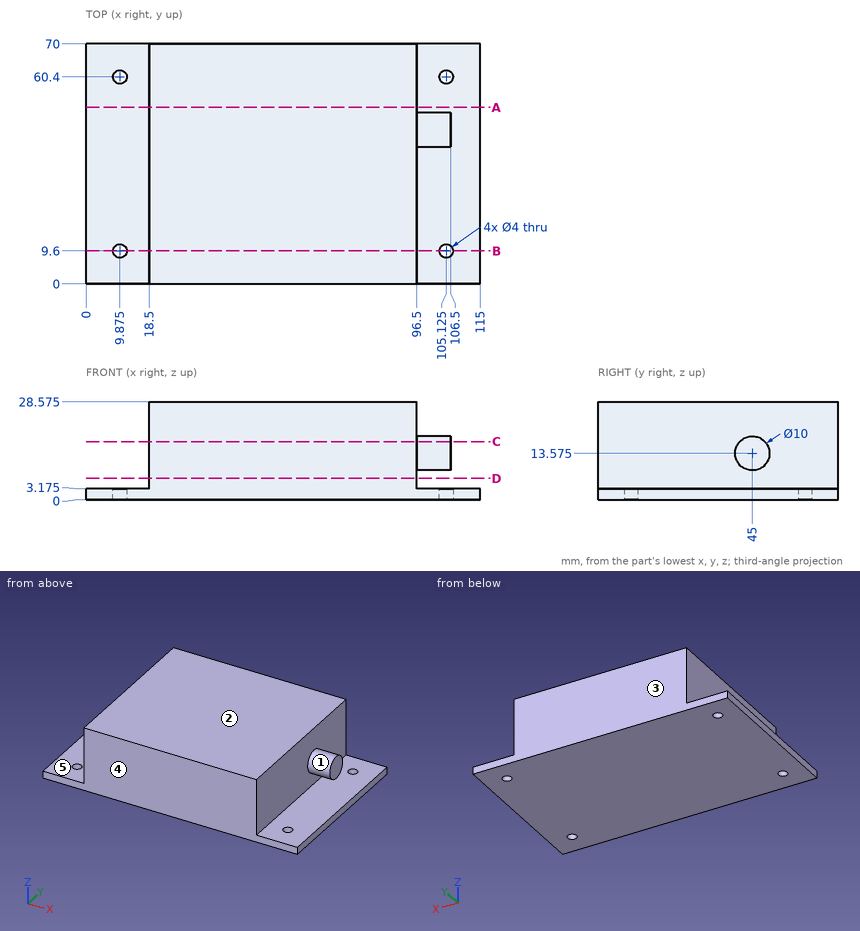
Here's the drawing with two shaded views (mm, measured from the low corner). I have some questions. A direction names the side the tool comes from. Give positions to 0.01 mm unless a question says otherwise; leave off trailing zeros. Order: outer loops, then holes, each group sorted by start corner. A loop starts at its lowest first (then second) coordinate and runs counter-clockwise, first axis right, second up. Notation, with made-up numbers: (81, 55.5) - (136, 55.5) arc R7 ccw to (136, 67.5) - close; hole circle Ø4 at (50, 69.25). An arc over 180 degrees is marked (long way). Use a Markdown table: item, result. Add a question column.
Q1. If we section it at A-A on y = 51.5: Write out the boundary of the cut face in (x, z) (3 decimals).
Q2. If we section it at B-B on y = 9.6: Write out the boundary of the cut face in (x, z) (3 decimals).
Q3. On a 3-axis mill with a long thin cutter (end or side, diameter ignored), from which of +Z, -Z, +X, -X, +Y, -Y can I reach the whole of each face in a straight line? I mean the marked faces 4 and 5. Say none if no direction works.
Q4. Please list where these lines run through material, in increasing order: line 1 along Z through (x, y) = (14.5, 9) (3 decimals); line 2 along X through (y, z) = (54, 18.5); line 3 along X through (y, z) = (43, 13).
Q5. If we mould it in two halves opening along Z, with no side actions, what happens to the marked faces 1, 2 and 3? For each: released by +Z, released by -Z, zero draft, split by the parting line, or undercut.
Q6. If we section it at D-D on z = 6.25: Write out the boundary of the cut face in (x, y), plus the area to 3 significant figures.
Q7. I'm going to push flat-ended pins straight in: pin 1 (20.5 mm diameter, centred on x = 108, y = 38, fed in from +Z) (3 decimals); pin 2 (12.5 mm diameter, centred on y = 41, z = 21, fed in from +X); pin 3 (5.5 mm diameter, centred on x = 11.5, y = 34.5, fed in from +Z) (3 decimals). Where does each tip first touch, or does it pass through?
Q8. If we section it at C-C on z = 17: Write out the boundary of the cut face in (x, y).
Answers follow:
| question | item | result |
|---|---|---|
| 1 | outline | (0, 0) - (115, 0) - (115, 3.175) - (96.5, 3.175) - (96.5, 28.575) - (18.5, 28.575) - (18.5, 3.175) - (0, 3.175) - close |
| 2 | outline | (0, 0) - (7.875, 0) - (7.875, 3.175) - (0, 3.175) - close; (11.875, 0) - (103.125, 0) - (103.125, 3.175) - (96.5, 3.175) - (96.5, 28.575) - (18.5, 28.575) - (18.5, 3.175) - (11.875, 3.175) - close; (107.125, 0) - (115, 0) - (115, 3.175) - (107.125, 3.175) - close |
| 3 | face 4 | +Z, -Z, +X, -X, -Y |
| 3 | face 5 | +Z, -X, +Y, -Y |
| 4 | line 1 | z = 0 to 3.175 |
| 4 | line 2 | x = 18.5 to 96.5 |
| 4 | line 3 | x = 18.5 to 106.5 |
| 5 | face 1 | undercut |
| 5 | face 2 | released by +Z |
| 5 | face 3 | zero draft |
| 6 | outline | (18.5, 0) - (96.5, 0) - (96.5, 70) - (18.5, 70) - close |
| 6 | area | 5,460 mm^2 |
| 7 | pin 1 | stops at z = 18.575 |
| 7 | pin 2 | stops at x = 106.5 |
| 7 | pin 3 | stops at z = 3.175 |
| 8 | outline | (18.5, 0) - (96.5, 0) - (96.5, 41.36) - (106.5, 41.36) - (106.5, 48.64) - (96.5, 48.64) - (96.5, 70) - (18.5, 70) - close |
